from build123d import *

# Parameters (mm, degrees)
SKETCH_1_R      = 4.75
EXTRUDE_1_DEPTH = 12.5
SKETCH_2_R      = 0.4
EXTRUDE_2_DEPTH = 2.5


with BuildPart() as part:
    # Эскиз1 → Бобышка-Вытянуть1 (new body)
    with BuildSketch(Plane.XY):
        with BuildLine():
            Line((12.25, -6.375), (-12.25, -6.375))
            Line((-12.25, -6.375), (-12.25, 6.375))
            ThreePointArc((-12.25, 6.375), (0, 18.625), (12.25, 6.375))
            Line((12.25, 6.375), (12.25, -6.375))
        make_face()
        with Locations((0, 6.375)):
            Circle(SKETCH_1_R, mode=Mode.SUBTRACT)
    extrude(amount=EXTRUDE_1_DEPTH)

    # Эскиз2 → Бобышка-Вытянуть2 (add)
    with BuildSketch(Plane.XZ.offset(6.375)):
        with Locations((7.4, 0.5)):
            Circle(SKETCH_2_R)
        with Locations((-7.4, 0.5)):
            Circle(SKETCH_2_R)
        with Locations((9.5, 12)):
            Circle(SKETCH_2_R)
        with Locations((-9.5, 12)):
            Circle(SKETCH_2_R)
    extrude(amount=EXTRUDE_2_DEPTH)


solid = part.part
Check sheet for the modelled part. Datum: model origin and axes. Units: mm. A direction names the side the tool comes from. Give positions to 0.01 mm unless a question says otherwise; leave off trailing zeros. Write each loop counter-clockwise with the first axis right and the second up, starting at its lowest first coordinate (ties: lowest second). Pieces come first, ordered by that corner, then holes. Notation, with made-up numbers: (23.25, -31.5) -> (76.25, -31.5) arc R9 ccw to (76.25, -14.5) -> close; hole circle Ø11 at (51, 20). An arc over 180 degrees is marked (long way). Write item = value, one per line.
Item 1: Tool access check on faces 5 (the cylindrical face through (-7.02, -7.61, 0.62)), 6 (the cylindrical face through (2.554, 10.38, 6.162)). Record the directions out of +Z, -Z, +X, -X, +Y, -Y that give a thin tool (end or side, any length) a straight path to the whole face; none if there is none.
Output:
face_5 = -Y
face_6 = +Z, -Z
Item 2: Scan lines: probe 1 along Y at (x, z) = (0, 3) (3 decimals); probe 2 along Y at (x, z) = (2, 6.75) (3 decimals); probe 3 along X at (y, z) = (6.25, 6.25). Record each from-to range of solid material in increasing order. Write a range as from..to.
Output:
probe_1 = -6.375..1.625, 11.125..18.625
probe_2 = -6.375..2.067, 10.683..18.461
probe_3 = -12.25..-4.75, 4.75..12.25
Item 3: Sectioned sample at A-A on x = 0. Record the boundary of the cut face in (y, z) (3 decimals).
Output:
outline = (-6.375, 0) -> (1.625, 0) -> (1.625, 12.5) -> (-6.375, 12.5) -> close; (11.125, 0) -> (18.625, 0) -> (18.625, 12.5) -> (11.125, 12.5) -> close
Item 4: Release check for a two-part mould opening along X. For faces 1 (the cylindrical face through (-9.315, -7.608, 11.645)), 2 (the cylindrical face through (-0.269, 18.622, 6.162)), 3 (the cylindrical face through (9.685, -7.608, 11.645)), 4 (the flat face through (-12.25, 0, 6)) record: +X half, -X half, draft (parallel to the pull), parting line (faces both ways), or undercut.
Output:
face_1 = undercut
face_2 = parting line
face_3 = undercut
face_4 = -X half
Item 5: Sectioned sample at B-B on z = 0.5. Record the boundary of the cut face in (x, y) (3 decimals), and give its area (3 significant figures).
Output:
outline = (-12.25, -6.375) -> (-7.8, -6.375) -> (-7.8, -8.875) -> (-7, -8.875) -> (-7, -6.375) -> (7, -6.375) -> (7, -8.875) -> (7.8, -8.875) -> (7.8, -6.375) -> (12.25, -6.375) -> (12.25, 6.375) arc R12.25 ccw to (-12.25, 6.375) -> close; hole circle Ø9.5 at (0, 6.375)
area = 481 mm^2
Item 6: Sectioned sample at D-D on x = -9.5. Record the boundary of the cut face in (y, z) (3 decimals), and give its area (3 significant figures).
Output:
outline = (-8.875, 11.6) -> (-6.375, 11.6) -> (-6.375, 0) -> (14.109, 0) -> (14.109, 12.5) -> (-6.375, 12.5) -> (-6.375, 12.4) -> (-8.875, 12.4) -> close
area = 258 mm^2
Item 7: Sectioned sample at C-C on y = 7.25. Record the boundary of the cut face in (x, z), and give its area (3 significant figures).
Output:
outline = (-12.22, 0) -> (-4.67, 0) -> (-4.67, 12.5) -> (-12.22, 12.5) -> close; (4.67, 0) -> (12.22, 0) -> (12.22, 12.5) -> (4.67, 12.5) -> close
area = 189 mm^2
Item 8: Gauge pin test, flat ends, axial feed: pin 1 (6 mm diameter, centred on x = 9.5, z = 9, fed in from +Y); pin 2 (1.5 mm diameter, centred on x = 9, z = 8, fed in from +Y); pin 3 (6 mm diameter, centred on y = 8, z = 8.5, fed in from +X); pin 4 (3 mm diameter, centred on y = 11.5, z = 4, fed in from -X). Record the tip position at first contact, or that the pin passes through.
Output:
pin_1 = 16.76
pin_2 = 15.43
pin_3 = 12.25
pin_4 = -11.7
